Autodesk Inventor part; units mm, degrees
ref_plane "YZ Plane" through (0, 0, 0) normal (1, 0, 0) x (0, 1, 0)
ref_plane "XZ Plane" through (0, 0, 0) normal (0, 1, 0) x (-1, 0, 0)
ref_plane "XY Plane" through (0, 0, 0) normal (0, 0, 1) x (1, 0, 0)
sketch "Sketch1" plane through (0, 0, 0) normal (0, 0, 1) x (1, 0, 0)
  circle A0 centre (0, 0) radius 15
  dimension "d0" = 30
extrude "Extrusion1" add sketch "Sketch1" along normal blind 4
sketch "Sketch2" plane through (0, 0, 4) normal (0, 0, 1) x (1, 0, 0)
  circle A0 centre (0, 0) radius 10 construction
  line L0 (0, 0) -> (-11.9207, 0) construction
  point P0 (-10, 0)
  point P1 (10, 0)
  dimension "d10" = 20
hole "Hole1" at (-10, 0, 4) at (10, 0, 4) direction (0, 0, -1) diameter 3.5 end through all counterbore diameter 6 counterbore depth 2
sketch "Sketch4" plane through (0, 0, 4) normal (0, 0, 1) x (1, 0, 0)
  arc A0 (-4.3301, 2.5) -> (4.3301, 2.5) centre (0, 0) ccw
  line L0 (-4.3301, 2.5) -> (4.3301, 2.5)
  circle A1 centre (10, 0) radius 3
  arc A2 (9.55, 2.9661) -> (9.55, -2.9661) centre (10, 0) ccw
  circle A3 centre (-10, 0) radius 3
  arc A4 (-9.5586, -2.9382) -> (-9.5586, 2.9382) centre (-10, 0) ccw
  arc A5 (-9.5586, -2.9382) -> (9.55, -2.9661) centre (0, 0) ccw
  arc A6 (9.55, 2.9661) -> (-9.5586, 2.9382) centre (0, 0) ccw
  point P0 (9.55, 2.9661)
  point P1 (-9.55, 2.9661)
  point P2 (-9.55, -2.9661)
  dimension "d12" = 10
  dimension "d13" = 2.5
  dimension "d14" = 10
  dimension "d15" = 10
extrude "Extrusion2" add sketch "Sketch4" along normal blind 15 contours A1 A5 A3 A6
equation "\"d15\" = d14"
properties part number "Motor-mount"
Could you check a few things on this model? Use its own coordinates, in mm. A direction names the side the tool comes from. Coordinates: 2 decimals unless noted, no trailing zeros. Order: outer loops, then holes, each group sorted by start corner. A loop starts at its lowest first (then second) coordinate and runs counter-clockwise, first axis right, second up. Notation, with made-up numbers: (82.5, 40.25) - (122.5, 40.25) arc R11 ccw to (122.5, 52.25) - close; hole circle Ø11 at (-10, -29.75). An arc over 180 degrees is marked (long way). Answer in a Markdown table with one row per item. Add a question column.
(1) If we mould it in two halves opening along Y, with no side actions, what happens to faces 1 (the face through (0, -5, 11)), 2 (the face through (0, 0, 0)), 3 (the face through (0, -10, 11))? For each: released by +Y, released by -Y, zero draft, split by the parting line, or undercut.
(2) Will these pins go through, and if not, where does the flat tip stop? pin 1 (5 mm diameter, centred on x = -10, y = 0, fed in from +Z); pin 2 (5 mm diameter, centred on x = -8, z = 16.5, fed in from +Y); pin 3 (3 mm diameter, centred on y = 10, z = 14.5, fed in from -X); pin 4 (3 mm diameter, centred on x = -10, y = 0, fed in from +Z).
(3) If we section it at C-C, the plane x = 10: Please give me the cut outline in (y, z), then the cut area to 3 significant figures.
(4) On a 3-axis mill with a long thin cutter (end or side, diameter ignored), from which of +Z, -Z, +X, -X, +Y, -Y can I reach the whole of each face in a straight line? I mean faces 4 (the face through (0, 10, 11)), 5 (the face through (-11.735, 0.228, 0.986)), 6 (the face through (0, 2.5, 11)). Say none if no direction works.
(5) If we section it at D-D, the plane z = 12: Please give me the cut outline in (x, y), then the cut area to 3 significant figures.
(6) If we section it at A-A, the plane x = 0: Please give me the cut outline in (y, z), then the cut area to 4 significant figures.
(7) If we section it at B-B, the plane y = -0.5: Please give me the cut outline in (x, z), then the cut area to 3 significant figures.
(8) I need wall thicknesses on L1, parallel to X at y = 0, z = 14; L2, parallel to Z at x = 7.75, y = -8; L3, parallel to X at y = 1, z = 3.75. Which ranges of each line are inside material? Lowest first, please.
Results are:
| question | item | result |
|---|---|---|
| 1 | face 1 | undercut |
| 1 | face 2 | zero draft |
| 1 | face 3 | released by -Y |
| 2 | pin 1 | stops at z = 2 |
| 2 | pin 2 | stops at y = 8.35 |
| 2 | pin 3 | stops at x = -5.27 |
| 2 | pin 4 | passes through |
| 3 | outline | (-11.18, 0) - (-1.75, 0) - (-1.75, 2) - (-3, 2) - (-3, 4) - (-11.18, 4) - close; (1.75, 0) - (11.18, 0) - (11.18, 4) - (3, 4) - (3, 2) - (1.75, 2) - close |
| 3 | area | 70.4 mm2 |
| 4 | face 4 | +Z, +Y |
| 4 | face 5 | +Z, -Z |
| 4 | face 6 | +Z |
| 5 | outline | (-9.55, -2.97) arc R10 ccw to (9.55, -2.97) arc R3 cw to (9.55, 2.97) arc R10 ccw to (-9.55, 2.97) arc R3 cw to start; hole (-4.33, 2.5) arc R5 ccw (long way) to (4.33, 2.5) - close |
| 5 | area | 225 mm2 |
| 6 | outline | (-15, 0) - (15, 0) - (15, 4) - (10, 4) - (10, 19) - (2.5, 19) - (2.5, 4) - (-5, 4) - (-5, 19) - (-10, 19) - (-10, 4) - (-15, 4) - close |
| 6 | area | 307.5 mm2 |
| 7 | outline | (-14.99, 0) - (-11.68, 0) - (-11.68, 2) - (-12.96, 2) - (-12.96, 4) - (-14.99, 4) - close; (-8.32, 0) - (8.32, 0) - (8.32, 2) - (7.04, 2) - (7.04, 19) - (4.97, 19) - (4.97, 4) - (-4.97, 4) - (-4.97, 19) - (-7.04, 19) - (-7.04, 2) - (-8.32, 2) - close; (11.68, 0) - (14.99, 0) - (14.99, 4) - (12.96, 4) - (12.96, 2) - (11.68, 2) - close |
| 7 | area | 145 mm2 |
| 8 | L1 | x = -7 to -5, 5 to 7 |
| 8 | L2 | z = 0 to 4 |
| 8 | L3 | x = -14.97 to -12.83, -7.17 to 7.17, 12.83 to 14.97 |
